Read the model definition and answer for the solid it produces. Units are mm, in the model's axes. A direction names the side the tool comes from. Give positions to 0.01 mm unless a question says otherwise; leave off trailing zeros. Order: outer loops, then holes, each group sorted by start corner. A loop starts at its lowest first (then second) coordinate and runs counter-clockwise, first axis right, second up. Notation, with made-up numbers: (7, -33.75) - (63, -33.75) arc R25 ccw to (63, -9.75) - close; hole circle Ø1 at (-23, 71). An arc over 180 degrees is marked (long way). Write each question's results on one line, items separated by ' | '. Start each with the question number.
Q1. Find section C-C on y = -7.5. Give the vertices of the cut face in (x, z), and give its area (3 significant figures).
Q2. A tool of negligible diameter and unlimited length cuts with its end or side. For faces 1 (the face through (-17.241, -5, 7)), 2 (the face through (-0.6, -5.07, 15.43)), from which of +Z, -Z, +X, -X, +Y, -Y can it reach the whole face along a straight path? Write none if from no direction.
Q3. Find section A-A on z = 4.5. Give the vertices of the cut face in (x, y), and give its area (3 significant figures).
Q4. A flat-ended cylindrical pin translates along its axis: P1, Ø8, axis at x = -4, z = 2.5, coming from the -Y side. Find the tip coordinate at first contact, or state that the pin passes through.
Q5. Find the intervals of material crossed by line 1 along Z through (x, y) = (-17, -2.75); line 2 along X through (y, z) = (-6.75, 7.5); line 3 along Y through (x, z) = (-11.5, 13), in increasing order. Write a range as from..to.
Q6. Find section B-B on x = -15.5. Give the vertices of the cut face in (y, z), and give its area (3 significant figures).
Q7. Find section D-D on x = -28. Give the vertices of the cut face in (y, z).
Q8. For a pull along Z with two mould halves and no side action, classify faces 3 (the face through (-17, -5, 16)), 4 (the face through (-11, -5, 10.502)), 5 (the face through (-28.54, -10.99, 7.06)) as +Z half, -Z half, draft (parallel to the pull), parting line (faces both ways), or undercut.
from build123d import *

# Parameters (mm, degrees)
F0_W     = 32
F0_H     = 16
F1_DEPTH = 10
F2_R     = 2.5
F3_DEPTH = 2
F4_R     = 2
F5_W     = 12
F5_H     = 7.054545
F6_DEPTH = 10


with BuildPart() as f1:
    # F0 (on Front) → F1 (new body)
    with BuildSketch(Plane.XZ):
        with Locations((-16, 8)):
            Rectangle(F0_W, F0_H)
    extrude(amount=F1_DEPTH)

    # F2 (on face) → F3 (join)
    with BuildSketch(Plane.XZ.offset(10)):
        with Locations((-28, 9.5)):
            Circle(F2_R)
    extrude(amount=F3_DEPTH)

    # F4
    f4_edges = [f1.edges().sort_by_distance(p)[0] for p in [
        (0, -5, 16),
    ]]
    fillet(f4_edges, radius=F4_R)

    # F5 (on face) → F6 (cut, through all)
    with BuildSketch(Plane.XZ.offset(10)):
        with Locations((-11.240668, 6.974615)):
            Rectangle(F5_W, F5_H)
    extrude(amount=-F6_DEPTH, mode=Mode.SUBTRACT)


solid = f1.part
Working result:
1) outline: (-32, 0) - (0, 0) - (0, 14) arc R2 ccw to (-2, 16) - (-32, 16) - close; hole (-17.24, 3.45) - (-5.24, 3.45) - (-5.24, 10.5) - (-17.24, 10.5) - close | area: 426 mm²
2) face 1: +Y, -Y | face 2: +Z, +X, +Y, -Y
3) outline: (-32, -10) - (-17.24, -10) - (-17.24, 0) - (-32, 0) - close; (-5.24, -10) - (0, -10) - (0, 0) - (-5.24, 0) - close | area: 200 mm²
4) P1: y = -10
5) line 1: 0..3.45, 10.5..16 | line 2: -32..-17.24, -5.24..0 | line 3: -10..0
6) outline: (-10, 0) - (0, 0) - (0, 3.45) - (-10, 3.45) - close; (-10, 10.5) - (0, 10.5) - (0, 16) - (-10, 16) - close | area: 89.5 mm²
7) outline: (-12, 7) - (-10, 7) - (-10, 0) - (0, 0) - (0, 16) - (-10, 16) - (-10, 12) - (-12, 12) - close
8) face 3: +Z half | face 4: undercut | face 5: parting line
